Could you check a few things on this model? Use its own coordinates, in mm. Face numbers are marked on the shaded views. A direction names the side the tool comes from. Give positions to 0.01 mm unless a question says otherwise; leave off trailing zeros. Loops run counter-clockwise (first coordinate to the right, second up) from the corner with the lowest first, then second, coordinate; pieces in that order, holes last. Notation, with made-up numbers: (16.25, 2.5) -> (37.25, 2.5) arc R17 cw to (37.25, 27.5) -> close; hole circle Ø9 at (65.5, 80.5). An arc over 180 degrees is marked (long way). Write each question's results on one line, items separated by ' | '. Start each with the question number.
Q1. If we section it at A-A, the plane y = 0: List the corners of the cut face in (x, z) for me.
Q2. Will these pins go through, and if not, where does the flat tip stop? P1, Ø8, axis at x = 99.5, y = 33, coming from the -Z side; P2, Ø12, axis at x = 171.5, z = 15, coming from the -Y side; P3, Ø2, axis at y = -2.5, z = 13.5, coming from the +X side.
Q3. If we section it at C-C, the plane x = 180: List the corners of the cut face in (y, z) for me, plus the area to 3 significant figures.
Q4. If we section it at D-D, the plane z = 58.5: List the corners of the cut face in (x, y) for me, plus the area to 3 significant figures.
Q5. Which directions (+Z, -Z, +X, -X, +Y, -Y) give clear straight access to the entire face, cutting with the end or side of a thin tool? Please do the marked faces 1, 2 and 3.
Q6. If we section it at B-B, the plane z = 25: List the corners of the cut face in (x, y) for me.
Q7. If I drill on line 1 along Z through (x, y) = (19, -39.5); line 2 along X through (y, z) = (1.5, 46.5); line 3 along X through (y, z) = (10, 31), over which ranges is the centre line in solid material (lowest first)?
from build123d import *

# Parameters (mm, degrees)
BOSS_EXTRUDE1_DEPTH = 50
SKETCH2_R           = 10
BOSS_EXTRUDE2_DEPTH = 20
SKETCH3_R           = 10
BOSS_EXTRUDE3_DEPTH = 20


with BuildPart() as part:
    # Sketch1 → Boss-Extrude1 (new body)
    with BuildSketch(Plane.XY):
        with BuildLine():
            Line((0, 60), (70, 60))
            Line((70, 60), (280, 30))
            Line((280, 30), (280, -30))
            Line((280, -30), (70, -60))
            Line((70, -60), (0, -60))
            ThreePointArc((0, -60), (-60, 0), (0, 60))
        make_face()
    extrude(amount=BOSS_EXTRUDE1_DEPTH)

    # Sketch2 → Boss-Extrude2 (add)
    with BuildSketch(Plane.XY.offset(50)):
        Circle(SKETCH2_R)
    extrude(amount=BOSS_EXTRUDE2_DEPTH)

    # Sketch3 → Boss-Extrude3 (add)
    with BuildSketch(Plane(origin=(280, 0, 0), x_dir=(0, 0, -1), z_dir=(1, 0, 0))):
        with Locations(Location((-25, 0, 0), (0, 0, 180))):
            Circle(SKETCH3_R)
    extrude(amount=BOSS_EXTRUDE3_DEPTH)


solid = part.part
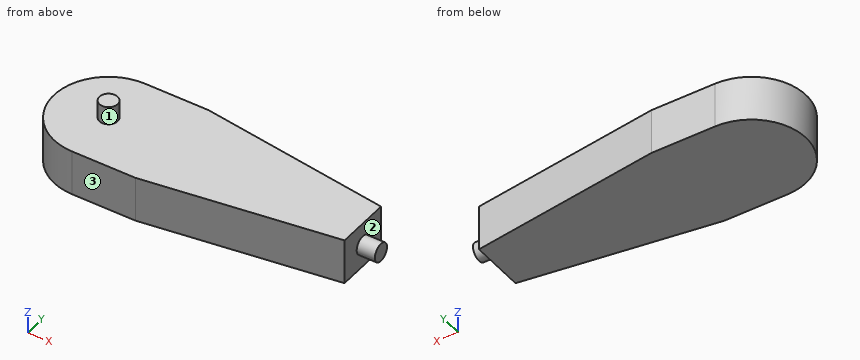
Final values:
1) outline: (-60, 0) -> (280, 0) -> (280, 15) -> (300, 15) -> (300, 35) -> (280, 35) -> (280, 50) -> (10, 50) -> (10, 70) -> (-10, 70) -> (-10, 50) -> (-60, 50) -> close
2) P1: stops at z = 0 | P2: stops at y = -46.36 | P3: stops at x = 280
3) outline: (-44.29, 0) -> (44.29, 0) -> (44.29, 50) -> (-44.29, 50) -> close | area: 4,430 mm²
4) outline: circle Ø20 at (0, 0) | area: 314 mm²
5) face 1: +Z | face 2: +X | face 3: +Z, -Z, +X, -X, -Y
6) outline: (0, -60) -> (70, -60) -> (280, -30) -> (280, -10) -> (300, -10) -> (300, 10) -> (280, 10) -> (280, 30) -> (70, 60) -> (0, 60) arc R60 ccw to start
7) line 1: z = 0 to 50 | line 2: x = -59.98 to 280 | line 3: x = -59.16 to 280
